```python
from build123d import *

# Parameters (mm, degrees)
ZAPAS_CZ_1_0_1_START        = 21.1
ZAPAS_CZ_1_0_1_DEPTH        = 8
WYTNIJ_WYCI_GNI_CIE1_DEPTH  = 393.717022804
DODANIE_WYCI_GNI_CIE1_DEPTH = 8


# Read off the part's stored shape, not the designer's step: Zapas-Część1.0-1
with BuildPart() as part:
    # Zapas-Część1.0-1 outline → Zapas-Część1.0-1 (new body)
    with BuildSketch(Plane(origin=(0, 0, 0), x_dir=(1, 0, 0), z_dir=(0, 1, 0)).offset(ZAPAS_CZ_1_0_1_START)):
        with BuildLine():
            ThreePointArc((-20.5, 21.6), (0, 1.1), (20.5, 21.6))
            Line((20.5, 21.6), (20.5, 371.6))
            ThreePointArc((20.5, 371.6), (0, 392.1), (-20.5, 371.6))
            Line((-20.5, 371.6), (-20.5, 21.6))
        make_face()
        with BuildLine():
            Line((-10, 64.6), (-10, 130.6))
            ThreePointArc((-10, 130.6), (0, 140.6), (10, 130.6))
            Line((10, 130.6), (10, 64.6))
            ThreePointArc((10, 64.6), (0, 54.6), (-10, 64.6))
        make_face(mode=Mode.SUBTRACT)
        with BuildLine():
            Line((-10, 164.6), (-10, 230.6))
            ThreePointArc((-10, 230.6), (0, 240.6), (10, 230.6))
            Line((10, 230.6), (10, 164.6))
            ThreePointArc((10, 164.6), (0, 154.6), (-10, 164.6))
        make_face(mode=Mode.SUBTRACT)
        with BuildLine():
            Line((-10, 264.6), (-10, 330.6))
            ThreePointArc((-10, 330.6), (0, 340.6), (10, 330.6))
            Line((10, 330.6), (10, 264.6))
            ThreePointArc((10, 264.6), (0, 254.6), (-10, 264.6))
        make_face(mode=Mode.SUBTRACT)
    extrude(amount=ZAPAS_CZ_1_0_1_DEPTH)

    # Szkic1 → Wytnij-wyciągnięcie1 (cut, through all)
    with BuildSketch(Plane(origin=(0, 29.1, 0), x_dir=(1, 0, 0), z_dir=(0, 1, 0))):
        with BuildLine():
            Line((-1.5, 23.6), (1.5, 23.6))
            ThreePointArc((1.5, 23.6), (0, 19.1), (-1.5, 23.6))
        make_face()
        with BuildLine():
            ThreePointArc((2.5, 371.6), (-1.118033989, 373.836067977), (-1.5, 369.6))
            ThreePointArc((-1.5, 369.6), (0, 369.1), (1.5, 369.6))
            ThreePointArc((1.5, 369.6), (2.236067977, 370.481966011), (2.5, 371.6))
        make_face()
    extrude(amount=-WYTNIJ_WYCI_GNI_CIE1_DEPTH, mode=Mode.SUBTRACT)

    # Szkic2 → Dodanie-wyciągnięcie1 (add)
    with BuildSketch(Plane(origin=(0, 29.1, 0), x_dir=(1, 0, 0), z_dir=(0, 1, 0))):
        with BuildLine():
            Line((-20.5, 371.6), (-20.5, 392.131331169))
            Line((-20.5, 392.131331169), (20.5, 392.131331169))
            Line((20.5, 392.131331169), (20.5, 371.6))
            Line((20.5, 371.6), (3.983153472, 371.6))
            Line((3.983153472, 371.6), (2.5, 371.6))
            ThreePointArc((2.5, 371.6), (0, 374.1), (-2.5, 371.6))
            Line((-2.5, 371.6), (-20.5, 371.6))
        make_face()
    extrude(amount=-DODANIE_WYCI_GNI_CIE1_DEPTH)


solid = part.part
```
CAD build for the part. Positions are in the model's coordinates, mm. A direction names the side the tool comes from. Round coordinates to 2 decimals unless told otherwise and drop trailing zeros. Order: outer loops, then holes, each group sorted by start corner. A loop starts at its lowest first (then second) coordinate and runs counter-clockwise, first axis right, second up. Notation, with made-up numbers: (-24, 79.25) - (15, 79.25) arc R18 cw to (15, 101.25) - close; hole circle Ø2 at (12, 73.25). An arc over 180 degrees is marked (long way). Use CSV: the item, a comma, the result in double quotes. Start each with the question number.
1) Saw through at C-C (z = -137). List the corners of the cut face in (x, y).
2) Saw through at B-B (y = 26.5). List the corners of the cut face in (x, z).
3) Pin check, flat tips, straight feed: pin 1 Ø3 at (x, z) = (0, -371.6) entering from -Y; pin 2 Ø2.5 at (x, y) = (-0.5, 26.5) entering from +Z. Stop position of each tip, or through.
4) Saw through at D-D (x = -17). List the corners of the cut face in (y, z), and give its area (3 significant figures).
5) Tool access for faces 1 (the flat face through (10, 25, -198)), 2 (the flat face through (20.5, 25, -209)): list every direction of +Z, -Z, +X, -X, +Y, -Y with a clear straight run to the whole face (end or side of a thin tool).
6) Wall check: L1, parallel to Z at x = 0, y = 23; L2, parallel to X at y = 24, z = -111; L3, parallel to X at y = 24, z = -371.6. Give the ranges that are in metal, low to high. Write a range as [from, to].
7) Saw through at A-A (z = -72). List the corners of the cut face in (x, y), and give its area (3 significant figures).
8) Two-plate mould, pull along X, no slides. Class faces 3 (the flat face through (10, 25, -98)), 4 (the flat face through (0, 25, -392.131)), 5 (the flat face through (-10, 25, -97)), 6 (the flat face through (-20.5, 25, -204)): pulls with the +X half, pulls with the -X half, needs draft (parallel to the pull), parting line crosses it, or undercut.
Values follow:
1,outline,"(-20.5, 21.1) - (-7.68, 21.1) - (-7.68, 29.1) - (-20.5, 29.1) - close; (7.68, 21.1) - (20.5, 21.1) - (20.5, 29.1) - (7.68, 29.1) - close"
2,outline,"(-20.5, -392.13) - (20.5, -392.13) - (20.5, -21.6) arc R20.5 ccw to (-20.5, -21.6) - close; hole (-10, -330.6) arc R10 ccw to (10, -330.6) - (10, -264.6) arc R10 ccw to (-10, -264.6) - close; hole (-10, -230.6) arc R10 ccw to (10, -230.6) - (10, -164.6) arc R10 ccw to (-10, -164.6) - close; hole (-10, -130.6) arc R10 ccw to (10, -130.6) - (10, -64.6) arc R10 ccw to (-10, -64.6) - close; hole circle Ø5 at (0, -371.6); hole (-1.5, -23.6) - (1.5, -23.6) arc R2.5 ccw (long way) to start"
3,pin 1,"passes through"
3,pin 2,"stops at z = -1.1"
4,outline,"(21.1, -392.13) - (29.1, -392.13) - (29.1, -10.14) - (21.1, -10.14) - close"
4,area,"3,060 mm2"
5,face 1,"+Y, -Y"
5,face 2,"+Z, -Z, +X, +Y, -Y"
6,L1,"z = [-392.13, -374.1], [-369.1, -340.6], [-254.6, -240.6], [-154.6, -140.6], [-54.6, -23.6], [-19.1, -1.1]"
6,L2,"x = [-20.5, -10], [10, 20.5]"
6,L3,"x = [-20.5, -2.5], [2.5, 20.5]"
7,outline,"(-20.5, 21.1) - (-10, 21.1) - (-10, 29.1) - (-20.5, 29.1) - close; (10, 21.1) - (20.5, 21.1) - (20.5, 29.1) - (10, 29.1) - close"
7,area,"168 mm2"
8,face 3,"undercut"
8,face 4,"needs draft"
8,face 5,"undercut"
8,face 6,"pulls with the -X half"
